```python
from build123d import *

# Parameters (mm, degrees)
F0_W         = 60
F0_H         = 2
F1_DEPTH     = 5
F2_W         = 9
F2_H         = 3
F3_DEPTH     = 5
F4_W         = 49
F4_H         = 3
F5_DEPTH     = 2.5
F6_T4_DEPTH  = 15.8584149398
F6_T9_DEPTH  = 28.7168298797
F6_T15_DEPTH = 28.7168298797
F6_T21_DEPTH = 15.8584149398


# Not quite as in the source:
# - a fillet or chamfer that OpenCascade refuses, or shapes differently, is made with other operations: its cross-section is extruded or revolved along the edge and cut away or added


with BuildPart() as f1:
    # F0 (on Top) → F1 (new body)
    with BuildSketch(Plane.XY):
        with BuildLine():
            ThreePointArc((21.3155073225, 23.6537444443), (19.7045946191, 27.5428317408), (15.8155073225, 29.1537444443))
            Line((15.8155073225, 29.1537444443), (15.8155073225, 25.6537444443))
            ThreePointArc((15.8155073225, 25.6537444443), (17.2297208849, 25.0679580066), (17.8155073225, 23.6537444443))
            ThreePointArc((17.8155073225, 23.6537444443), (17.2297208849, 22.2395308819), (15.8155073225, 21.6537444443))
            Line((15.8155073225, 21.6537444443), (15.8155073225, 18.1537444443))
            ThreePointArc((15.8155073225, 18.1537444443), (19.7045946191, 19.7646571477), (21.3155073225, 23.6537444443))
        make_face()
        with BuildLine():
            Line((15.8155073225, 29.1537444443), (14.120912728, 28.8861768767))
            ThreePointArc((14.120912728, 28.8861768767), (11.3674588589, 26.8886887815), (10.3155073225, 23.6537444443))
            Line((10.3155073225, 23.6537444443), (13.8155073225, 23.6537444443))
            ThreePointArc((13.8155073225, 23.6537444443), (14.4012937602, 25.0679580066), (15.8155073225, 25.6537444443))
            Line((15.8155073225, 25.6537444443), (15.8155073225, 29.1537444443))
        make_face()
        with BuildLine():
            Line((13.8155073225, 23.6537444443), (10.3155073225, 23.6537444443))
            ThreePointArc((10.3155073225, 23.6537444443), (11.3674588589, 20.418800107), (14.120912728, 18.4213120118))
            Line((14.120912728, 18.4213120118), (15.8155073225, 18.1537444443))
            Line((15.8155073225, 18.1537444443), (15.8155073225, 21.6537444443))
            ThreePointArc((15.8155073225, 21.6537444443), (14.4012937602, 22.2395308819), (13.8155073225, 23.6537444443))
        make_face()
        with BuildLine():
            Line((14.120912728, 28.8861768767), (9.8155073225, 28.2063760232))
            Line((9.8155073225, 28.2063760232), (9.8155073225, 24.6537444443))
            Line((9.8155073225, 24.6537444443), (9.8155073225, 23.6537444443))
            Line((9.8155073225, 23.6537444443), (10.3155073225, 23.6537444443))
            ThreePointArc((10.3155073225, 23.6537444443), (11.3674588589, 26.8886887815), (14.120912728, 28.8861768767))
        make_face()
        with BuildLine():
            Line((10.3155073225, 23.6537444443), (9.8155073225, 23.6537444443))
            Line((9.8155073225, 23.6537444443), (9.8155073225, 22.6537444443))
            Line((9.8155073225, 22.6537444443), (9.8155073225, 19.1011128653))
            Line((9.8155073225, 19.1011128653), (14.120912728, 18.4213120118))
            ThreePointArc((14.120912728, 18.4213120118), (11.3674588589, 20.418800107), (10.3155073225, 23.6537444443))
        make_face()
        with Locations((-23.6844926775, 23.6537444443)):
            Rectangle(F0_W, F0_H)
        Polygon((9.8155073225, 24.6537444443), (6.3155073225, 24.6537444443), (6.3155073225, 22.6537444443), (9.8155073225, 22.6537444443), (9.8155073225, 23.6537444443), align=None)
        with BuildLine():
            ThreePointArc((-57.6844926775, 23.6537444443), (-58.7364442138, 26.8886887815), (-61.4898980829, 28.8861768767))
            Line((-61.4898980829, 28.8861768767), (-63.1844926775, 29.1537444443))
            Line((-63.1844926775, 29.1537444443), (-63.1844926775, 25.6537444443))
            ThreePointArc((-63.1844926775, 25.6537444443), (-61.7702791151, 25.0679580066), (-61.1844926775, 23.6537444443))
            Line((-61.1844926775, 23.6537444443), (-57.6844926775, 23.6537444443))
        make_face()
        with BuildLine():
            ThreePointArc((-61.4898980829, 18.4213120118), (-58.7364442138, 20.418800107), (-57.6844926775, 23.6537444443))
            Line((-57.6844926775, 23.6537444443), (-61.1844926775, 23.6537444443))
            ThreePointArc((-61.1844926775, 23.6537444443), (-61.7702791151, 22.2395308819), (-63.1844926775, 21.6537444443))
            Line((-63.1844926775, 21.6537444443), (-63.1844926775, 18.1537444443))
            Line((-63.1844926775, 18.1537444443), (-61.4898980829, 18.4213120118))
        make_face()
        with BuildLine():
            Line((-63.1844926775, 25.6537444443), (-63.1844926775, 29.1537444443))
            ThreePointArc((-63.1844926775, 29.1537444443), (-68.6844926775, 23.6537444443), (-63.1844926775, 18.1537444443))
            Line((-63.1844926775, 18.1537444443), (-63.1844926775, 21.6537444443))
            ThreePointArc((-63.1844926775, 21.6537444443), (-65.1844926775, 23.6537444443), (-63.1844926775, 25.6537444443))
        make_face()
        with BuildLine():
            Line((-57.1844926775, 24.6537444443), (-57.1844926775, 28.2063760232))
            Line((-57.1844926775, 28.2063760232), (-61.4898980829, 28.8861768767))
            ThreePointArc((-61.4898980829, 28.8861768767), (-58.7364442138, 26.8886887815), (-57.6844926775, 23.6537444443))
            Line((-57.6844926775, 23.6537444443), (-57.1844926775, 23.6537444443))
            Line((-57.1844926775, 23.6537444443), (-57.1844926775, 24.6537444443))
        make_face()
        with BuildLine():
            Line((-57.1844926775, 22.6537444443), (-57.1844926775, 23.6537444443))
            Line((-57.1844926775, 23.6537444443), (-57.6844926775, 23.6537444443))
            ThreePointArc((-57.6844926775, 23.6537444443), (-58.7364442138, 20.418800107), (-61.4898980829, 18.4213120118))
            Line((-61.4898980829, 18.4213120118), (-57.1844926775, 19.1011128653))
            Line((-57.1844926775, 19.1011128653), (-57.1844926775, 22.6537444443))
        make_face()
        Polygon((-53.6844926775, 22.6537444443), (-53.6844926775, 24.6537444443), (-57.1844926775, 24.6537444443), (-57.1844926775, 23.6537444443), (-57.1844926775, 22.6537444443), align=None)
    extrude(amount=F1_DEPTH)

    # F2 (on face) → F3 (join)
    with BuildSketch(Plane(origin=(0, 0, 0), x_dir=(1, 0, 0), z_dir=(0, 0, -1))):
        with Locations((5.3155073225, -21.1537444443)):
            Rectangle(F2_W, F2_H)
        with Locations((5.3155073225, -26.1537444443)):
            Rectangle(F2_W, F2_H)
        with Locations((-52.6844926775, -21.1537444443)):
            Rectangle(F2_W, F2_H)
        with Locations((-52.6844926775, -26.1537444443)):
            Rectangle(F2_W, F2_H)
    extrude(amount=-F3_DEPTH)

    # F4 (on face) → F5 (join)
    with BuildSketch(Plane.XY.offset(5)):
        with Locations((-23.6844926775, 21.1537444443)):
            Rectangle(F4_W, F4_H)
        with Locations((-23.6844926775, 26.1537444443)):
            Rectangle(F4_W, F4_H)
    extrude(amount=-F5_DEPTH)

    # F6: chamfer of 5 on 2 edges, made by hand


with BuildPart() as f6_tool2:
    # F6_s3 → F6_t4 (new body)
    with BuildSketch(Plane.XZ.offset(-6.7953295044)):
        Polygon((0.8155073225, 5), (5.8155073225, 0), (0.8155073225, 0), align=None)
    extrude(amount=-F6_T4_DEPTH)

    split(bisect_by=Plane.XY.offset(2.5), keep=Keep.BOTTOM)


with BuildPart() as f1_1:
    add(f1.part)

    # F6_t1: cut F6_tool2
    add(f6_tool2.part, mode=Mode.SUBTRACT)


with BuildPart() as f6_tool7:
    # F6_s8 → F6_t9 (new body)
    with BuildSketch(Plane.XZ.offset(-6.7953295044)):
        Polygon((0.8155073225, 5), (5.8155073225, 0), (0.8155073225, 0), align=None)
    extrude(amount=-F6_T9_DEPTH)

    split(bisect_by=Plane.XY.offset(2.5), keep=Keep.BOTTOM)

    split(bisect_by=Plane.XZ.offset(-24.6537444443), keep=Keep.BOTTOM)


with BuildPart() as f1_2:
    add(f1_1.part)

    # F6_t6: cut F6_tool7
    add(f6_tool7.part, mode=Mode.SUBTRACT)


with BuildPart() as f6_tool13:
    # F6_s14 → F6_t15 (new body)
    with BuildSketch(Plane.XZ.offset(-11.7953295044)):
        Polygon((0.8155073225, 5), (5.8155073225, 0), (0.8155073225, 0), align=None)
    extrude(amount=-F6_T15_DEPTH)

    split(bisect_by=Plane.XZ.offset(-22.6537444443), keep=Keep.TOP)

    split(bisect_by=Plane.XY.offset(2.5), keep=Keep.BOTTOM)


with BuildPart() as f1_3:
    add(f1_2.part)

    # F6_t12: cut F6_tool13
    add(f6_tool13.part, mode=Mode.SUBTRACT)


with BuildPart() as f6_tool19:
    # F6_s20 → F6_t21 (new body)
    with BuildSketch(Plane.XZ.offset(-24.6537444443)):
        Polygon((0.8155073225, 5), (5.8155073225, 0), (0.8155073225, 0), align=None)
    extrude(amount=-F6_T21_DEPTH)

    split(bisect_by=Plane.XY.offset(2.5), keep=Keep.BOTTOM)


with BuildPart() as f1_4:
    add(f1_3.part)

    # F6_t18: cut F6_tool19
    add(f6_tool19.part, mode=Mode.SUBTRACT)


solid = f1_4.part
```
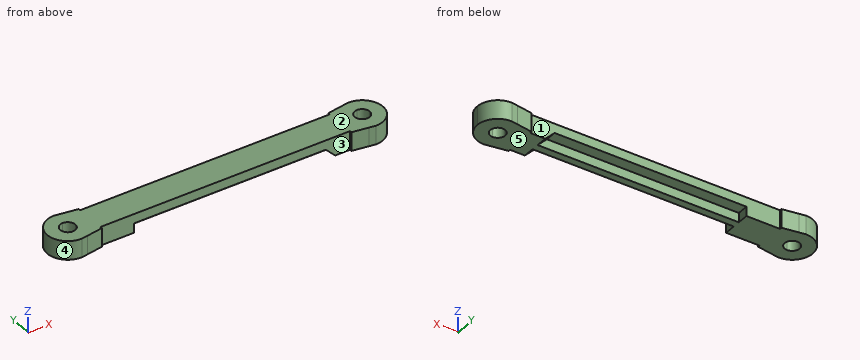
For this review, take the finished solid that the model builds, in its own axes (mm). Face numbers are marked on the shaded views. A direction names the side the tool comes from. Give positions to 0.01 mm unless a question says otherwise; leave off trailing zeros. Order: outer loops, then holes, each group sorted by start corner. A loop starts at its lowest first (then second) coordinate and runs counter-clockwise, first axis right, second up.
1) Take a section at B-B (z = 1.3). Give the boundary of the cut face in (x, y), then the cut area to 3 significant figures.
2) Insertion check: pin 1 (1.5 mm diameter, centred on x = -37, z = 2, fed in from +Y); pin 2 (1.2 mm diameter, centred on y = 26.5, z = 2, fed in from +X); pin 3 (0.8 mm diameter, centred on x = -32.5, z = 2, fed in from -Y). Each pin has a flat end and moves straight along its axis. Give the tip position at first contact, or say it passes through.
3) For the marked faces 1 and 2, list the 3-axis set-ups (+Z, -Z, +X, -X, +Y, -Y) from which the entire face can be reached by the end or side of a thin tool; tool diameter is ignored.
4) Take a section at C-C (x = 12). Give the boundary of the cut face in (y, z).
5) Take a section at A-A (x = -1). Give the boundary of the cut face in (y, z).
6) The part is to be moulded in two halves that separate along X. For the marked faces 3, 4 and 5, say which applies: released by +X, released by -X, zero draft, split by the parting line, or undercut.
7) Wall thickness on line 1 (X direction, y = 23.5, z = 4.6); line 2 (X direction, y = 24.5, z = 4.1); line 3 (Y direction, x = -34, z = 2.9): over which ranges is each line inside the solid? List them lowest first.
Derived:
1. outline: (-63.18, 18.15) - (-57.18, 19.1) - (-57.18, 19.65) - (-48.18, 19.65) - (-48.18, 22.65) - (4.52, 22.65) - (4.52, 19.65) - (9.82, 19.65) - (9.82, 19.1) - (15.82, 18.15) arc R5.5 ccw to (15.82, 29.15) - (9.82, 28.21) - (9.82, 27.65) - (4.52, 27.65) - (4.52, 24.65) - (-48.18, 24.65) - (-48.18, 27.65) - (-57.18, 27.65) - (-57.18, 28.21) - (-63.18, 29.15) arc R5.5 ccw to start; hole circle Ø4 at (-63.18, 23.65); hole circle Ø4 at (15.82, 23.65)
1. area: 410 mm2
2. pin 1: stops at y = 27.65
2. pin 2: stops at x = 20.84
2. pin 3: stops at y = 22.65
3. face 1: +Z, -Z, +Y
3. face 2: +Z, +X, -X, +Y, -Y
4. outline: (18.76, 0) - (28.55, 0) - (28.55, 5) - (18.76, 5) - close
5. outline: (19.65, 2.5) - (22.65, 2.5) - (22.65, 0) - (24.65, 0) - (24.65, 2.5) - (27.65, 2.5) - (27.65, 5) - (19.65, 5) - close
6. face 3: undercut
6. face 4: released by -X
6. face 5: zero draft
7. line 1: x = -68.68 to -65.18, -61.19 to 13.82, 17.81 to 21.31
7. line 2: x = -68.62 to -65, -61.37 to 14, 17.63 to 21.25
7. line 3: y = 19.65 to 27.65
